Design review of the part built by this model. Coordinates are the model's own, in mm. Face numbers are marked on the shaded views. A direction names the side the tool comes from. Round coordinates to 2 decimals unless told otherwise and drop trailing zeros. Order: outer loops, then holes, each group sorted by start corner. A loop starts at its lowest first (then second) coordinate and runs counter-clockwise, first axis right, second up. Notation, with made-up numbers: (19.5, 25) - (73.5, 25) arc R15 ccw to (73.5, 35) - close; hole circle Ø2 at (-32.75, -12.75). An arc over 180 degrees is marked (long way). Write item = value, one per line.
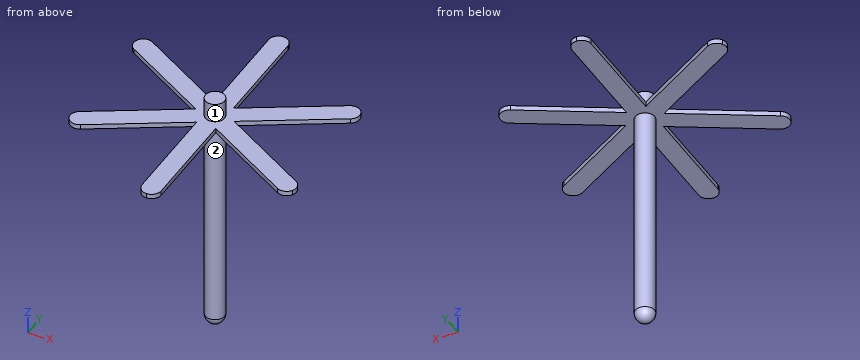
from build123d import *

# Parameters (mm, degrees)
F0_R     = 10.16
F1_DEPTH = 263.398
F4_DEPTH = 5.08
F5_R     = 10.16


with BuildPart() as f1:
    # F0 (on Top) → F1 (new body)
    with BuildSketch(Plane.XY):
        Circle(F0_R)
    extrude(amount=F1_DEPTH)

    # F3 (on offset) → F4 (join)
    with BuildSketch(Plane.XY.offset(237.998)):
        with BuildLine():
            ThreePointArc((0, 136.525), (-7.184205, 133.549205), (-10.16, 126.365))
            Line((-10.16, 126.365), (-10.16, 17.597636))
            Line((-10.16, 17.597636), (-104.3553, 71.981318))
            ThreePointArc((-104.3553, 71.981318), (-112.064902, 72.996306), (-118.234118, 68.2625))
            ThreePointArc((-118.234118, 68.2625), (-119.249107, 60.552899), (-114.5153, 54.383682))
            Line((-114.5153, 54.383682), (-20.32, 0))
            Line((-20.32, 0), (-114.5153, -54.383682))
            ThreePointArc((-114.5153, -54.383682), (-119.249107, -60.552899), (-118.234118, -68.2625))
            ThreePointArc((-118.234118, -68.2625), (-112.064902, -72.996306), (-104.3553, -71.981318))
            Line((-104.3553, -71.981318), (-10.16, -17.597636))
            Line((-10.16, -17.597636), (-10.16, -126.365))
            ThreePointArc((-10.16, -126.365), (-7.184205, -133.549205), (0, -136.525))
            ThreePointArc((0, -136.525), (7.184205, -133.549205), (10.16, -126.365))
            Line((10.16, -126.365), (10.16, -17.597636))
            Line((10.16, -17.597636), (104.3553, -71.981318))
            ThreePointArc((104.3553, -71.981318), (112.064902, -72.996306), (118.234118, -68.2625))
            ThreePointArc((118.234118, -68.2625), (119.249107, -60.552899), (114.5153, -54.383682))
            Line((114.5153, -54.383682), (20.32, 0))
            Line((20.32, 0), (114.5153, 54.383682))
            ThreePointArc((114.5153, 54.383682), (119.249107, 60.552899), (118.234118, 68.2625))
            ThreePointArc((118.234118, 68.2625), (112.064902, 72.996306), (104.3553, 71.981318))
            Line((104.3553, 71.981318), (10.16, 17.597636))
            Line((10.16, 17.597636), (10.16, 126.365))
            ThreePointArc((10.16, 126.365), (7.184205, 133.549205), (0, 136.525))
        make_face()
    extrude(amount=F4_DEPTH)

    # F5
    f5_edges = [f1.edges().sort_by_distance(p)[0] for p in [
        (-10.16, 0, 0),
    ]]
    fillet(f5_edges, radius=F5_R)


solid = f1.part
Item 1: Insertion check: P1, Ø5, axis at x = 46, y = 24.5, coming from the -Z side; P2, Ø2.5, axis at y = 72.5, z = 241, coming from the -X side; P3, Ø2.5, axis at y = -46, z = 241, coming from the -X side. Each pin has a flat end and moves straight along its axis. Give the tip position at first contact, or say it passes through.
Data:
P1 = 238
P2 = -115.61
P3 = -102.16
Item 2: For the marked faces 1 and 2, list the 3-axis set-ups (+Z, -Z, +X, -X, +Y, -Y) from which the entire face can be reached by the end or side of a thin tool; tool diameter is ignored.
Data:
face_1 = +Z
face_2 = -Z
Item 3: For line 1 along X through (y, z) = (-23.5, 241); line 2 along Z through (x, y) = (16.5, -2.5); line 3 along Y through (x, z) = (-42.5, 240), list the stretches that pass through material, from the lowest coordinate up. Write a range as [from, to].
Data:
line_1 = [-61.02, -20.38], [-10.16, 10.16], [20.38, 61.02]
line_2 = [238, 243.08]
line_3 = [-36.27, -12.81], [12.81, 36.27]
Item 4: Take a section at B-B, the plane x = -29. State the section outline as (y, z) points.
Data:
outline = (-28.47, 238) - (-5.01, 238) - (-5.01, 243.08) - (-28.47, 243.08) - close; (5.01, 238) - (28.47, 238) - (28.47, 243.08) - (5.01, 243.08) - close
Item 5: Take a section at A-A, the plane y = 22. State the section outline as (x, z) points, and give its area (3 significant figures).
Data:
outline = (-58.43, 238) - (-17.79, 238) - (-17.79, 243.08) - (-58.43, 243.08) - close; (-10.16, 238) - (10.16, 238) - (10.16, 243.08) - (-10.16, 243.08) - close; (17.79, 238) - (58.43, 238) - (58.43, 243.08) - (17.79, 243.08) - close
area = 516 mm2
Item 6: Take a section at D-D, the plane z = 70. State the section outline as (x, y) points.
Data:
outline = circle Ø20.32 at (0, 0)
Item 7: Take a section at C-C, the plane x = 6. State the section outline as (y, z) points.
Data:
outline = (-134.56, 238) - (-8.2, 238) - (-8.2, 10.16) arc R8.2 ccw to (8.2, 10.16) - (8.2, 238) - (134.56, 238) - (134.56, 243.08) - (8.2, 243.08) - (8.2, 263.4) - (-8.2, 263.4) - (-8.2, 243.08) - (-134.56, 243.08) - close
